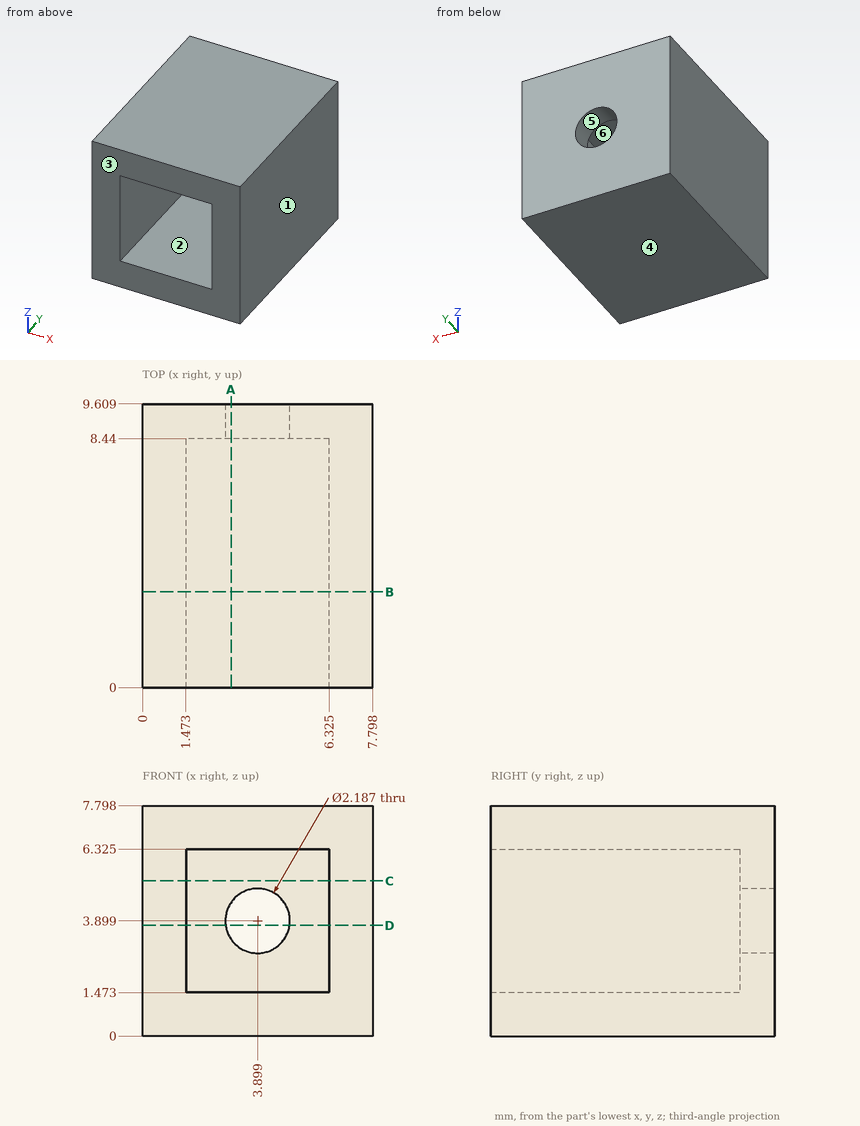
Design review of the part shown in the three views and the two pictorial views. Dimensions are in mm from the part's minimum x, y and z. A direction names the side the tool comes from. Give positions to 0.01 mm unless a question says otherwise; leave off trailing zeros. Write each loop counter-clockwise with the first axis right and the second up, starting at its lowest first coordinate (ties: lowest second). Pieces come first, ordered by that corner, then holes. Notation, with made-up numbers: (29.5, 53.5) -> (33.5, 53.5) arc R28 cw to (33.5, 86.5) -> close; hole circle Ø3 at (39.5, 78). An arc over 180 degrees is marked (long way). Answer in a Markdown table with one row per item.
1) Add section A-A on x = 3. State the section outline as (y, z) points (1 decimal).
Worked answers:
| item | result |
|---|---|
| outline | (0, 0) -> (9.6, 0) -> (9.6, 3.3) -> (8.4, 3.3) -> (8.4, 1.5) -> (0, 1.5) -> close; (0, 6.3) -> (8.4, 6.3) -> (8.4, 4.5) -> (9.6, 4.5) -> (9.6, 7.8) -> (0, 7.8) -> close |
2) Add section D-D on z = 3.75. State the section outline as (x, y) points (1 decimal).
Worked answers:
| item | result |
|---|---|
| outline | (0, 0) -> (1.5, 0) -> (1.5, 8.4) -> (2.8, 8.4) -> (2.8, 9.6) -> (0, 9.6) -> close; (5, 8.4) -> (6.3, 8.4) -> (6.3, 0) -> (7.8, 0) -> (7.8, 9.6) -> (5, 9.6) -> close |
3) For L1, parallel to X at y = 3.5, z = 2 (1 decimal); L2, parallel to Y at x = 5, z = 4.25, list the stretches that pass through material, from the lowest coordinate up. Write a range as [from, to].
Worked answers:
| item | result |
|---|---|
| L1 | [0, 1.5], [6.3, 7.8] |
| L2 | [8.44, 9.61] |
4) Mouldability with a two-part tool opening along Z and no side actions: class the marked faces 3, 4, 5 and 6 as +Z half, -Z half, draft (parallel to the pull), parting line (faces both ways), or undercut.
Worked answers:
| item | result |
|---|---|
| face 3 | draft |
| face 4 | -Z half |
| face 5 | undercut |
| face 6 | undercut |
5) Add section B-B on y = 3.25. State the section outline as (x, z) points (1 decimal).
Worked answers:
| item | result |
|---|---|
| outline | (0, 0) -> (7.8, 0) -> (7.8, 7.8) -> (0, 7.8) -> close; hole (1.5, 1.5) -> (6.3, 1.5) -> (6.3, 6.3) -> (1.5, 6.3) -> close |
6) Add section C-C on z = 5.25. State the section outline as (x, y) points (1 decimal).
Worked answers:
| item | result |
|---|---|
| outline | (0, 0) -> (1.5, 0) -> (1.5, 8.4) -> (6.3, 8.4) -> (6.3, 0) -> (7.8, 0) -> (7.8, 9.6) -> (0, 9.6) -> close |
7) Tool access review of the marked faces 1 and 2: name each direction out of +Z, -Z, +X, -X, +Y, -Y from which nothing blocks a thin tool from reaching the whole face with its end or side.
Worked answers:
| item | result |
|---|---|
| face 1 | +Z, -Z, +X, +Y, -Y |
| face 2 | -Y |
8) Clearance check with a flat-ended pin moving along its axis: P1, Ø1.5, axis at x = 2.5, z = 4.5, coming from the -Y side. State where the tip first meets the part, or that it passes through.
Worked answers:
| item | result |
|---|---|
| P1 | y = 8.44 |
